Input: part model. Units: mm. Frame: model coordinates. Face numbers are marked on the shaded views. A direction names the side the tool comes from. Give positions to 0.01 mm unless a question says otherwise; leave off trailing zeros. Loops run counter-clockwise (first coordinate to the right, second up) from the corner with the lowest first, then second, coordinate; pieces in that order, holes last. Notation, with made-up numbers: M -7.75,30.25 L 25.25,30.25 A22 ccw 25.25,47.25 Z; hole C 41,-4.75 d1. An arc over 180 degrees is marked long. One line per item, written item: value. Start each with the question number.
(1) Pull-direction query (Z, two-part tool) for the marked faces 1, 2 and 3; classes: released by +Z, released by -Z, zero draft, split by the parting line, or undercut.
(2) Section B-B on x = 5.75. Output: boundary loops of the cut face in (y, z).
(3) Section C-C on y = 1.2. Output: boundary loops of the cut face in (x, z), plus the area to 3 significant figures.
(4) Pin query (flat end, axial travel): P1, Ø4, axis at x = -1.5, z = 1, coming from the +Y side; P2, Ø1, axis at y = 2.5, z = -2.5, coming from the +X side; P3, Ø5.5, axis at x = 0, z = 0, coming from the +Y side; P4, Ø1, axis at x = -2, y = 2.5, coming from the -Z side. Return the tip coordinate at first contact, or that it passes through.
(5) Section A-A on z = 0. Output: boundary loops of the cut face in (x, y), plus the area to 3 significant figures.
(6) Section D-D on z = 6.75. Output: boundary loops of the cut face in (x, y), plus the area to 3 significant figures.
(7) Access query for the marked faces 4 and 5. Directions: +Z, -Z, +X, -X, +Y, -Y. A direction counts if a zero-diameter tool reaches every point of the face in a straight line with its end or side. Return the directions, or none.
(8) Ray query, line 1 along X through (y, z) = (1.95, 0); line 2 along X through (y, z) = (2.25, 0); line 3 along X through (y, z) = (3.65, 0). Return the intervals inside material, ascending. Write a range as from..to.
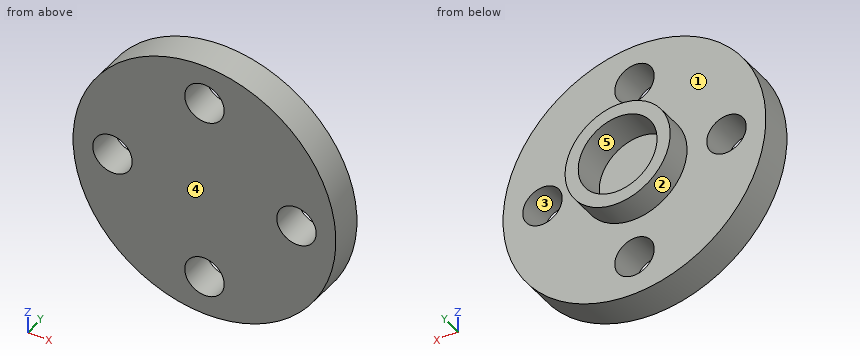
```python
from build123d import *

# Parameters (mm, degrees)
SKETCH1_R                      = 10
BOSS_EXTRUDE1_DEPTH            = 2.5
SKETCH2_R                      = 4
SKETCH2_R_2                    = 3
BOSS_EXTRUDE2_DEPTH            = 2
CUT_EXTRUDE1_START             = -0.5
SKETCH3_R                      = 3
CUT_EXTRUDE1_DEPTH             = 0.5
CUT_EXTRUDE3_REACH             = 16.361
SKETCH4_R                      = 1.5
CUT_EXTRUDE3_DIRECTION_2_DEPTH = 15.361406616


with BuildPart() as part:
    # Sketch1 → Boss-Extrude1 (new body)
    with BuildSketch(Plane(origin=(0, 0, 0), x_dir=(1, 0, 0), z_dir=(0, 1, 0))):
        with Locations(Location((0, 0, 0), (0, 0, 270))):
            Circle(SKETCH1_R)
    extrude(amount=BOSS_EXTRUDE1_DEPTH)

    # Sketch2 → Boss-Extrude2 (add)
    with BuildSketch(Plane(origin=(0, 2.5, 0), x_dir=(1, 0, 0), z_dir=(0, 1, 0))):
        with Locations(Location((0, 0, 0), (0, 0, 270))):
            Circle(SKETCH2_R)
        with Locations(Location((0, 0, 0), (0, 0, 270))):
            Circle(SKETCH2_R_2, mode=Mode.SUBTRACT)
    extrude(amount=BOSS_EXTRUDE2_DEPTH)

    # Sketch3 → Cut-Extrude1 (cut)
    with BuildSketch(Plane(origin=(0, 2.5, 0), x_dir=(1, 0, 0), z_dir=(0, 1, 0)).offset(CUT_EXTRUDE1_START)):
        with Locations(Location((0, 0, 0), (0, 0, 270))):
            Circle(SKETCH3_R)
    extrude(amount=CUT_EXTRUDE1_DEPTH, mode=Mode.SUBTRACT)

    # Sketch4 → Cut-Extrude3 (cut, up to next)
    with BuildSketch(Plane(origin=(0, 2, 0), x_dir=(1, 0, 0), z_dir=(0, 1, 0)), mode=Mode.PRIVATE) as cut_extrude3_sk1:
        with Locations(Location((0, 7, 0), (0, 0, 270))):
            Circle(SKETCH4_R)
    cut_extrude3_tool1 = extrude(cut_extrude3_sk1.sketch, amount=-CUT_EXTRUDE3_REACH, mode=Mode.PRIVATE) & part.part
    # Sketch4 → Cut-Extrude3 (cut, up to next)
    with BuildSketch(Plane(origin=(0, 2, 0), x_dir=(1, 0, 0), z_dir=(0, 1, 0)), mode=Mode.PRIVATE) as cut_extrude3_sk2:
        with Locations(Location((7, 0, 0), (0, 0, 270))):
            Circle(SKETCH4_R)
    cut_extrude3_tool2 = extrude(cut_extrude3_sk2.sketch, amount=-CUT_EXTRUDE3_REACH, mode=Mode.PRIVATE) & part.part
    # Sketch4 → Cut-Extrude3 (cut, up to next)
    with BuildSketch(Plane(origin=(0, 2, 0), x_dir=(1, 0, 0), z_dir=(0, 1, 0)), mode=Mode.PRIVATE) as cut_extrude3_sk3:
        with Locations(Location((0, -7, 0), (0, 0, 270))):
            Circle(SKETCH4_R)
    cut_extrude3_tool3 = extrude(cut_extrude3_sk3.sketch, amount=-CUT_EXTRUDE3_REACH, mode=Mode.PRIVATE) & part.part
    # Sketch4 → Cut-Extrude3 (cut, up to next)
    with BuildSketch(Plane(origin=(0, 2, 0), x_dir=(1, 0, 0), z_dir=(0, 1, 0)), mode=Mode.PRIVATE) as cut_extrude3_sk4:
        with Locations(Location((-7, 0, 0), (0, 0, 270))):
            Circle(SKETCH4_R)
    cut_extrude3_tool4 = extrude(cut_extrude3_sk4.sketch, amount=-CUT_EXTRUDE3_REACH, mode=Mode.PRIVATE) & part.part
    add(cut_extrude3_tool1.solids().sort_by_distance((0, 2, -7))[0], mode=Mode.SUBTRACT)
    add(cut_extrude3_tool2.solids().sort_by_distance((7, 2, 0))[0], mode=Mode.SUBTRACT)
    add(cut_extrude3_tool3.solids().sort_by_distance((0, 2, 7))[0], mode=Mode.SUBTRACT)
    add(cut_extrude3_tool4.solids().sort_by_distance((-7, 2, 0))[0], mode=Mode.SUBTRACT)

    # Sketch4 → Cut-Extrude3 direction 2 (cut)
    with BuildSketch(Plane(origin=(0, 2, 0), x_dir=(1, 0, 0), z_dir=(0, 1, 0))):
        with Locations(Location((0, 7, 0), (0, 0, 270))):
            Circle(SKETCH4_R)
        with Locations(Location((7, 0, 0), (0, 0, 270))):
            Circle(SKETCH4_R)
        with Locations(Location((0, -7, 0), (0, 0, 270))):
            Circle(SKETCH4_R)
        with Locations(Location((-7, 0, 0), (0, 0, 270))):
            Circle(SKETCH4_R)
    extrude(amount=CUT_EXTRUDE3_DIRECTION_2_DEPTH, mode=Mode.SUBTRACT)


solid = part.part
```
Output values:
1. face 1: zero draft
1. face 2: split by the parting line
1. face 3: undercut
2. outline: M 0,-8.18 L 2.5,-8.18 L 2.5,-0.83 L 0,-0.83 Z; M 0,0.83 L 2.5,0.83 L 2.5,8.18 L 0,8.18 Z
3. outline: C 0,0 d20; hole C -7,0 d3; hole C 0,-7 d3; hole C 0,7 d3; hole C 7,0 d3
3. area: 286 mm²
4. P1: stops at y = 4.5
4. P2: stops at x = 9.8
4. P3: stops at y = 2
4. P4: stops at z = -9.89
5. outline: M -10,0 L -8.5,0 L -8.5,2.5 L -10,2.5 Z; M -5.5,0 L 5.5,0 L 5.5,2.5 L 4,2.5 L 4,4.5 L 3,4.5 L 3,2 L -3,2 L -3,4.5 L -4,4.5 L -4,2.5 L -5.5,2.5 Z; M 8.5,0 L 10,0 L 10,2.5 L 8.5,2.5 Z
5. area: 36.0 mm²
6. outline: M -7.38,0 L -1.48,0 L -1.48,2.5 L -7.38,2.5 Z; M 1.48,0 L 7.38,0 L 7.38,2.5 L 1.48,2.5 Z
6. area: 29.5 mm²
7. face 4: +Z, -Z, +X, -X, -Y
7. face 5: +Y
8. line 1: x = -10..-8.5, -5.5..5.5, 8.5..10
8. line 2: x = -10..-8.5, -5.5..-3, 3..5.5, 8.5..10
8. line 3: x = -4..-3, 3..4
